Source: CAD feature listing. Evaluate the final solid. Frame: model axes, mm. A direction names the side the tool comes from. Give positions to 0.01 mm unless a question says otherwise; leave off trailing zeros. Loops run counter-clockwise (first coordinate to the right, second up) from the corner with the lowest first, then second, coordinate; pieces in that order, holes last. Notation, with made-up numbers: (57.25, 28) -> (67.25, 28) arc R28 cw to (67.25, 49) -> close; hole circle Ø2 at (89, -1). An arc over 180 degrees is marked (long way). Put each result on its own line as item: value.
```python
from build123d import *

# Parameters (mm, degrees)
SKIZZE1_W                            = 20
SKIZZE1_H                            = 20
SKIZZE1_R                            = 6
AUFSATZ_LINEAR_AUSTRAGEN1_DEPTH      = 40
SKIZZE2_R                            = 1
SKIZZE2_R_2                          = 1.75
SCHNITT_LINEAR_AUSTRAGEN1_DEPTH      = 3
SKIZZE3_R                            = 0.5
SCHNITT_LINEAR_AUSTRAGEN2_DEPTH      = 2
SCHNITT_LINEAR_AUSTRAGEN3_REACH      = 46.989
SCHNITT_LINEAR_AUSTRAGEN3_END_RADIUS = 6
SKIZZE4_R                            = 3.25
F_7_0_7_DURCHMESSER_BOHRUNG1_REACH   = 32
F_7_0_7_DURCHMESSER_BOHRUNG1_BORE_R  = 3.5
M2_GEWINDEBOHRUNG1_REACH             = 39.417
M2_GEWINDEBOHRUNG1_BORE_R            = 0.8


with BuildPart() as part:
    # Skizze1 → Aufsatz-Linear austragen1 (new body)
    with BuildSketch(Plane.XY):
        Rectangle(SKIZZE1_W, SKIZZE1_H)
        Circle(SKIZZE1_R, mode=Mode.SUBTRACT)
    extrude(amount=AUFSATZ_LINEAR_AUSTRAGEN1_DEPTH)

    # Skizze2 → Schnitt-Linear austragen1 (cut)
    with BuildSketch(Plane.XZ.offset(10)):
        with Locations(Location((0, 30, 0), (0, 0, 270))):
            Circle(SKIZZE2_R)
        with Locations(Location((0, 10, 0), (0, 0, 270))):
            Circle(SKIZZE2_R)
        with Locations(Location((0, 20, 0), (0, 0, 270))):
            Circle(SKIZZE2_R_2)
    extrude(amount=-SCHNITT_LINEAR_AUSTRAGEN1_DEPTH, mode=Mode.SUBTRACT)

    # Skizze3 → Schnitt-Linear austragen2 (cut)
    with BuildSketch(Plane.XZ.offset(7)):
        with Locations(Location((0, 30, 0), (0, 0, 270))):
            Circle(SKIZZE3_R)
        with Locations(Location((0, 10, 0), (0, 0, 270))):
            Circle(SKIZZE3_R)
    extrude(amount=-SCHNITT_LINEAR_AUSTRAGEN2_DEPTH, mode=Mode.SUBTRACT)

    # Schnitt-Linear austragen3: up to this cylinder (the profile starts outside it)
    schnitt_linear_austragen3_end = Plane(origin=(0, 0, 20), z_dir=(0, 0, -1)) * Cylinder(SCHNITT_LINEAR_AUSTRAGEN3_END_RADIUS, 106.978, mode=Mode.PRIVATE)
    # Skizze4 → Schnitt-Linear austragen3 (cut, up to the surface)
    with BuildSketch(Plane(origin=(0, -8, 0), x_dir=(-1, 0, 0), z_dir=(0, -1, 0)), mode=Mode.PRIVATE) as schnitt_linear_austragen3_sk1:
        with Locations(Location((0, -20, 0), (0, 0, 90))):
            Circle(SKIZZE4_R)
    schnitt_linear_austragen3_tool1 = extrude(schnitt_linear_austragen3_sk1.sketch, amount=-SCHNITT_LINEAR_AUSTRAGEN3_REACH, mode=Mode.PRIVATE) - schnitt_linear_austragen3_end
    add(schnitt_linear_austragen3_tool1.solids().sort_by_distance((0, -8, 20))[0], mode=Mode.SUBTRACT)

    # Ø7.0 (7) Durchmesser Bohrung1 bore (on position points) → Ø7.0 (7) Durchmesser Bohrung1 (cut, up to next)
    with BuildSketch(Plane(origin=(0, 10, 20), x_dir=(0, 0, 1), z_dir=(0, 1, 0)), mode=Mode.PRIVATE) as f_7_0_7_durchmesser_bohrung1_sk1:
        Circle(F_7_0_7_DURCHMESSER_BOHRUNG1_BORE_R)
    f_7_0_7_durchmesser_bohrung1_tool1 = extrude(f_7_0_7_durchmesser_bohrung1_sk1.sketch, amount=-F_7_0_7_DURCHMESSER_BOHRUNG1_REACH, mode=Mode.PRIVATE) & part.part
    add(f_7_0_7_durchmesser_bohrung1_tool1.solids().sort_by_distance((0, 10, 20))[0], mode=Mode.SUBTRACT)

    # M2 Gewindebohrung1 bore (on position points) → M2 Gewindebohrung1 (cut, up to next)
    with BuildSketch(Plane(origin=(0, 10, 30), x_dir=(0, 0, 1), z_dir=(0, 1, 0)), mode=Mode.PRIVATE) as m2_gewindebohrung1_sk1:
        Circle(M2_GEWINDEBOHRUNG1_BORE_R)
    m2_gewindebohrung1_tool1 = extrude(m2_gewindebohrung1_sk1.sketch, amount=-M2_GEWINDEBOHRUNG1_REACH, mode=Mode.PRIVATE) & part.part
    # M2 Gewindebohrung1 bore (on position points) → M2 Gewindebohrung1 (cut, up to next)
    with BuildSketch(Plane(origin=(0, 10, 30), x_dir=(0, 0, 1), z_dir=(0, 1, 0)), mode=Mode.PRIVATE) as m2_gewindebohrung1_sk2:
        with Locations((-20, 0)):
            Circle(M2_GEWINDEBOHRUNG1_BORE_R)
    m2_gewindebohrung1_tool2 = extrude(m2_gewindebohrung1_sk2.sketch, amount=-M2_GEWINDEBOHRUNG1_REACH, mode=Mode.PRIVATE) & part.part
    add(m2_gewindebohrung1_tool1.solids().sort_by_distance((0, 10, 30))[0], mode=Mode.SUBTRACT)
    add(m2_gewindebohrung1_tool2.solids().sort_by_distance((0, 10, 10))[0], mode=Mode.SUBTRACT)


solid = part.part
```
(1) Draft query along X for faces 1 (the flat face through (2, -10, 20)), 2 (the cylindrical face through (-2.883, -6.871, 18.5)), 3 (the flat face through (10, 0, 20)). Return one class per face: released by +X, released by -X, zero draft, split by the parting line, or undercut.
Calculated:
face 1: zero draft
face 2: undercut
face 3: released by +X
(2) First-contact query: P1, Ø3, axis at x = 0, z = 20, coming from the +Y side; P2, Ø1.6, axis at x = 0, z = 10, coming from the -Y side. Flat tips, straight axial feed; report the tip coordinate or a pass-through.
Calculated:
P1: passes through
P2: stops at y = -7
(3) Section D-D on x = 4.5. Return loops of the section in (y, z), then the cut area to 3 significant figures.
Calculated:
outline: (-10, 0) -> (-3.97, 0) -> (-3.97, 40) -> (-10, 40) -> close; (3.97, 0) -> (10, 0) -> (10, 40) -> (3.97, 40) -> close
area: 483 mm²
(4) Section B-B on x = 2.25. Return loops of the section in (y, z), then the cut area to 3 significant figures.
Calculated:
outline: (-10, 0) -> (-5.56, 0) -> (-5.56, 17.65) -> (-8, 17.65) -> (-8, 22.35) -> (-5.56, 22.35) -> (-5.56, 40) -> (-10, 40) -> close; (5.56, 0) -> (10, 0) -> (10, 17.32) -> (5.56, 17.32) -> close; (5.56, 22.68) -> (10, 22.68) -> (10, 40) -> (5.56, 40) -> close
area: 320 mm²
(5) Section C-C on z = 20. Return loops of the section in (x, y).
Calculated:
outline: (-10, -10) -> (-1.75, -10) -> (-1.75, -8) -> (-3.25, -8) -> (-3.25, -5.04) arc R6 cw to (-3.5, 4.87) -> (-3.5, 10) -> (-10, 10) -> close; (1.75, -10) -> (10, -10) -> (10, 10) -> (3.5, 10) -> (3.5, 4.87) arc R6 cw to (3.25, -5.04) -> (3.25, -8) -> (1.75, -8) -> close
(6) Line query: probe 1 along Z at (x, y) = (0, 7.5); probe 2 along Z at (x, y) = (0, -6.3); probe 3 along X at (y, z) = (-8, 10). Output: solid intervals per line, ascending. Write a range as from..to.
Calculated:
probe 1: z = 0..9.2, 10.8..16.5, 23.5..29.2, 30.8..40
probe 2: z = 0..9.5, 10.5..16.75, 23.25..29.5, 30.5..40
probe 3: x = -10..-1, 1..10
(7) Section A-A on y = 0. Return loops of the section in (x, z).
Calculated:
outline: (-10, 0) -> (-6, 0) -> (-6, 40) -> (-10, 40) -> close; (6, 0) -> (10, 0) -> (10, 40) -> (6, 40) -> close
(8) Reachability of faces 4 (the cylindrical face through (-6, 0, 20)), 5 (the cylindrical face through (0, -9, 29)), 6 (the cylindrical face through (-2.1, 7.5, 17.2)) from +Z, -Z, +X, -X, +Y, -Y: full face, straight path, thin tool, end or side. Return the list, or none.
Calculated:
face 4: +Z, -Z
face 5: -Y
face 6: +Y
